Check sheet for the drawn part. Datum: minimum x, y, z corner. Units: mm. A direction names the side the tool comes from. Give positions to 0.01 mm unless a question says otherwise; leave off trailing zeros. Order: outer loops, then holes, each group sorted by start corner. A loop starts at its lowest first (then second) coordinate and runs counter-clockwise, first axis right, second up. Notation, with made-up numbers: M 55,18 L 90,18 A9 ccw 90,27 Z; hole C -10,-19 d1. An arc over 180 degrees is marked long. One line per question, with ' | ' between items. Start each with the question number.
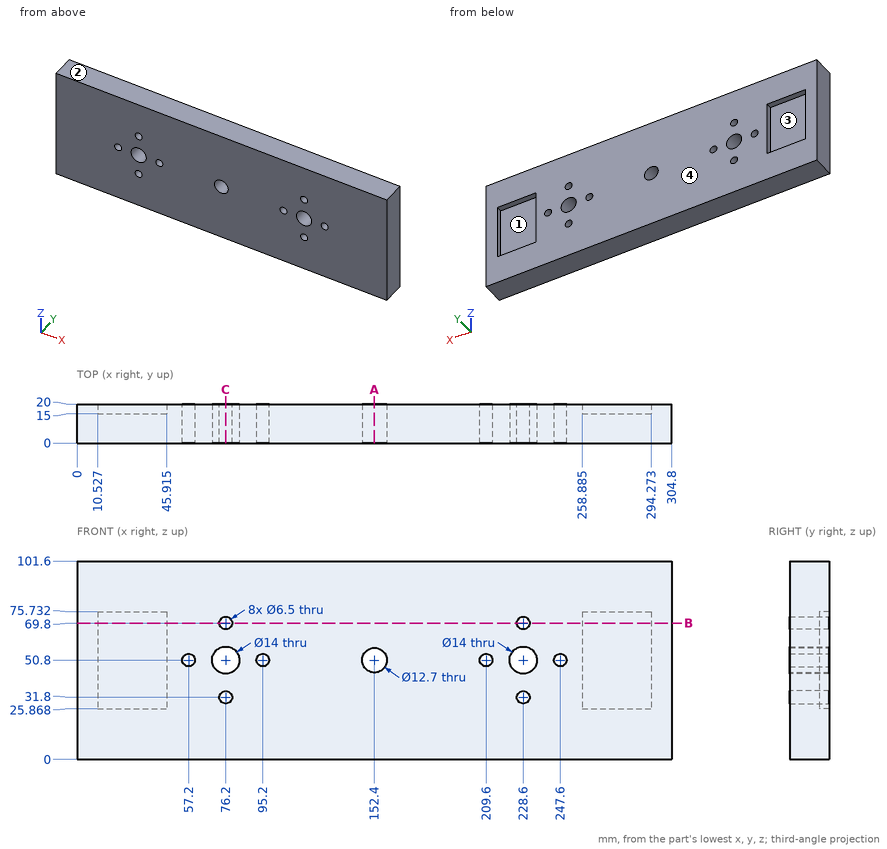
Item 1: Section check C-C, the plane x = 76.2. Record the cut outline in (y, z), then the cut area to 3 significant figures.
Item 2: Set-up check for the marked faces 3 and 4: record each of +Z, -Z, +X, -X, +Y, -Y from which the full face is reachable in a straight line by a thin tool's end or side.
Item 3: Section check A-A, the plane x = 152.4. Record the cut outline in (y, z).
Item 4: Draft check along X on the marked faces 1 and 2. Enter one of: released by +X, released by -X, zero draft, split by the parting line, or undercut.
Item 5: Section check B-B, the plane z = 69.8. State how many separate pieces and enclosed holes the cut face has, then the cut area to 3 significant figures.
Item 6: Scan lines: probe 1 along X at (y, z) = (9.5, 31.8); probe 2 along X at (y, z) = (16.25, 42) (1 decimal); probe 3 along Z at (x, y) = (57.2, 12). Record each from-to range of solid material in increasing order. Write a range as [from, to].
Item 7: Go/stop test with flat-tipped pins: P1, Ø17.5, axis at x = 277.5, z = 57, coming from the +Y side; P2, Ø6, axis at x = 228.6, z = 69.8, coming from the -Y side. Record where each tip stops, or that it passes through.
Reported:
1) outline: M 0,0 L 20,0 L 20,28.55 L 0,28.55 Z; M 0,35.05 L 20,35.05 L 20,43.8 L 0,43.8 Z; M 0,57.8 L 20,57.8 L 20,66.55 L 0,66.55 Z; M 0,73.05 L 20,73.05 L 20,101.6 L 0,101.6 Z | area: 1,490 mm^2
2) face 3: +Y | face 4: +Z, -Z, +X, -X, +Y
3) outline: M 0,0 L 20,0 L 20,44.45 L 0,44.45 Z; M 0,57.15 L 20,57.15 L 20,101.6 L 0,101.6 Z
4) face 1: undercut | face 2: zero draft
5) separate pieces: 3 | enclosed holes: 0 | area: 5,480 mm^2
6) probe 1: x = [0, 72.95], [79.45, 225.35], [231.85, 304.8] | probe 2: x = [0, 10.5], [45.9, 258.9], [294.3, 304.8] | probe 3: z = [0, 47.55], [54.05, 101.6]
7) P1: stops at y = 15 | P2: passes through
